```python
from build123d import *

# Parameters (mm, degrees)
SKETCH14_R          = 16.9
BOSS_EXTRUDE1_DEPTH = 82
CHAMFER1_SIZE       = 2


with BuildPart() as part:
    # Sketch14 → Boss-Extrude1 (new body)
    with BuildSketch(Plane(origin=(0, 0, 0), x_dir=(0, 0, -1), z_dir=(1, 0, 0))):
        Circle(SKETCH14_R)
    extrude(amount=BOSS_EXTRUDE1_DEPTH)

    # Sketch16 → Cut-Revolve4 (revolve, cut)
    with BuildSketch(Plane(origin=(0, 0, 0), x_dir=(1, 0, 0), z_dir=(0, 1, 0))):
        Polygon((1.414213562, 16.9), (1.414213562, 0), (0, 0), (0, 15.485786438), align=None)
    revolve(axis=Axis((82, 0, 0), (-1, 0, 0)), mode=Mode.SUBTRACT)


with BuildPart() as body_2:
    # of the pieces the cut leaves, the one that is kept (cut_revolve4_keep)
    add(part.part.solids().sort_by_distance((82, 0, -16.9))[0])

    # Chamfer1
    chamfer1_edges = [body_2.edges().sort_by_distance(p)[0] for p in [
        (82, 0, 16.9),
        (1.414213562, 0, 16.9),
    ]]
    chamfer(chamfer1_edges, length=CHAMFER1_SIZE)


solid = body_2.part
```
The listing builds one solid part. Answer for the finished solid, in the listing's coordinates (mm). Coordinates: 2 decimals unless noted, no trailing zeros. Write each loop counter-clockwise with the first axis right and the second up, starting at its lowest first coordinate (ties: lowest second). Pieces come first, ordered by that corner, then holes. Notation, with made-up numbers: M -33.5,20 L -25.5,20 A24 cw -25.5,39 Z; hole C -19.75,10 d6. An arc over 180 degrees is marked long. Use a Markdown table: item, result. Add a question column.
1. Section A-A (x = 25) is taken. Give the vertices of the cut face in (y, z), plus the area to 3 significant figures.
2. Straight lines are drawn through the part: line 1 along Z through (x, y) = (5, 13.5); line 2 along Y through (x, z) = (67.5, -8.5); line 3 along Y through (x, z) = (17, 6). For each, find the intervals that lie inside material, in ascending order. Write a range as [from, to].
3. Given P1, Ø1, axis at x = 22.5, y = -5, coming from the -Z side; P2, Ø1.5, axis at x = 74, y = 7, coming from the -Z side; P3, Ø4, axis at x = 12.5, z = -3, coming from the +Y side, each flat-ended and moving along its own axis, determine where each tip first touches the part or whether it passes through.
Data:
| question | item | result |
|---|---|---|
| 1 | outline | C 0,0 d33.8 |
| 1 | area | 897 mm2 |
| 2 | line 1 | z = [-10.17, 10.17] |
| 2 | line 2 | y = [-14.61, 14.61] |
| 2 | line 3 | y = [-15.8, 15.8] |
| 3 | P1 | stops at z = -16.29 |
| 3 | P2 | stops at z = -15.7 |
| 3 | P3 | stops at y = 16.87 |
